Design review of the part built by this model. Coordinates are the model's own, in mm. A direction names the side the tool comes from. Give positions to 0.01 mm unless a question says otherwise; leave off trailing zeros. Loops run counter-clockwise (first coordinate to the right, second up) from the corner with the lowest first, then second, coordinate; pieces in that order, holes last. Notation, with made-up numbers: (-21.75, 59) -> (-10.75, 59) arc R27 cw to (-10.75, 80) -> close; hole circle Ø5 at (-34, 64.5). An arc over 180 degrees is marked (long way). Answer in a Markdown table with one row per item. Add a question column.
(1) For pin 1 (12 mm diameter, centred on x = -23.5, y = -8.5, fed in from -Z); pin 2 (3 mm diameter, centred on x = -5, z = 1.5, fed in from -Y); pin 3 (2.5 mm diameter, centred on x = 45.72, y = 0, fed in from -Z); pin 4 (3 mm diameter, centred on y = 4.5, z = 3, fed in from -X), all flat-tipped, find the tip position at first contact; note any pin that passes through.
(2) For faces 4 (the cylindrical face through (-44.29, 0.45, 2.88)), 5 (the flat face through (12.7, 6, 3)), list the 3-axis set-ups (+Z, -Z, +X, -X, +Y, -Y) from which the entire face can be reached by the end or side of a thin tool; tool diameter is ignored.
(3) Consider section C-C on z = 2.15. Count the separate pieces of the cut face and the enclosed holes in it, then the cut area to 3 significant figures.
(4) Consider section D-D on y = 22.86. Write out the cut boundary in (x, z), then the cut area to 3 significant figures.
(5) Consider section A-A on y = -45.72. Write out the cut boundary in (x, z).
(6) For line 1 (Y direction, x = 0, z = 1.4); line 2 (Y direction, x = 2.5, z = 3.6); line 3 (X direction, y = 17.5, z = 5), list the stretches that pass through material, from the lowest coordinate up.
(7) Consider section B-B on x = -22. Write out the cut boundary in (y, z).
(8) Draft analysis for pull direction Y (two halves, no side actions). For faces 1 (the flat face through (-12.7, 6, 3)), 2 (the cylindrical face through (0.279, -12.697, 2.88)), 3 (the cylindrical face through (-38.83, -24.32, 2.88)), state which applies: +Y half, -Y half, draft (parallel to the pull), parting line (faces both ways), or undercut.
from build123d import *

# Parameters (mm, degrees)
SKETCH1_R           = 3
SKETCH1_R_2         = 1.5
SKETCH1_R_3         = 1.65
BOSS_EXTRUDE1_DEPTH = 5.842
FILLET1_R           = 18


with BuildPart() as part:
    # Sketch1 → Boss-Extrude1 (new body)
    with BuildSketch(Plane.XY):
        with BuildLine():
            Line((-12.7, 0), (-12.7, 49.186888497))
            ThreePointArc((-12.7, 49.186888497), (0, -50.8), (12.7, 49.186888497))
            Line((12.7, 49.186888497), (12.7, 0))
            ThreePointArc((12.7, 0), (0, -12.7), (-12.7, 0))
        make_face()
        with Locations((22, 0)):
            Circle(SKETCH1_R, mode=Mode.SUBTRACT)
        with Locations((0, -22)):
            Circle(SKETCH1_R, mode=Mode.SUBTRACT)
        with Locations((-22, 0)):
            Circle(SKETCH1_R, mode=Mode.SUBTRACT)
        with Locations((-45.72, 0)):
            Circle(SKETCH1_R_2, mode=Mode.SUBTRACT)
        with Locations((45.72, 0)):
            Circle(SKETCH1_R_2, mode=Mode.SUBTRACT)
        with Locations((0, -45.72)):
            Circle(SKETCH1_R_2, mode=Mode.SUBTRACT)
        with Locations((39.594681461, 22.86)):
            Circle(SKETCH1_R_3, mode=Mode.SUBTRACT)
        with Locations((39.594681461, -22.86)):
            Circle(SKETCH1_R_3, mode=Mode.SUBTRACT)
        with Locations((-39.594681461, -22.86)):
            Circle(SKETCH1_R_3, mode=Mode.SUBTRACT)
        with Locations((-39.594681461, 22.86)):
            Circle(SKETCH1_R_3, mode=Mode.SUBTRACT)
    extrude(amount=BOSS_EXTRUDE1_DEPTH)

    # Fillet1
    fillet1_edges = [part.edges().sort_by_distance(p)[0] for p in [
        (12.7, 49.186888497, 2.921),
        (-12.7, 49.186888497, 2.921),
    ]]
    fillet(fillet1_edges, radius=FILLET1_R)


solid = part.part
Values follow:
| question | item | result |
|---|---|---|
| 1 | pin 1 | z = 0 |
| 1 | pin 2 | y = -50.68 |
| 1 | pin 3 | through |
| 1 | pin 4 | x = -50.71 |
| 2 | face 4 | +Z, -Z |
| 2 | face 5 | +Z, -Z, +Y |
| 3 | separate pieces | 1 |
| 3 | enclosed holes | 10 |
| 3 | area | 5,550 mm2 |
| 4 | outline | (-44.7, 0) -> (-41.24, 0) -> (-41.24, 5.84) -> (-44.7, 5.84) -> close; (-37.94, 0) -> (-16.7, 0) -> (-16.7, 5.84) -> (-37.94, 5.84) -> close; (16.7, 0) -> (37.94, 0) -> (37.94, 5.84) -> (16.7, 5.84) -> close; (41.24, 0) -> (44.7, 0) -> (44.7, 5.84) -> (41.24, 5.84) -> close |
| 4 | area | 289 mm2 |
| 5 | outline | (-22.14, 0) -> (-1.5, 0) -> (-1.5, 5.84) -> (-22.14, 5.84) -> close; (1.5, 0) -> (22.14, 0) -> (22.14, 5.84) -> (1.5, 5.84) -> close |
| 6 | line 1 | -50.8 to -47.22, -44.22 to -25, -19 to -12.7 |
| 6 | line 2 | -50.74 to -23.66, -20.34 to -12.45 |
| 6 | line 3 | -47.69 to -13.71, 13.71 to 47.69 |
| 7 | outline | (-45.79, 0) -> (-3, 0) -> (-3, 5.84) -> (-45.79, 5.84) -> close; (3, 0) -> (27.31, 0) -> (27.31, 5.84) -> (3, 5.84) -> close |
| 8 | face 1 | draft |
| 8 | face 2 | +Y half |
| 8 | face 3 | undercut |
